Work out the finished part from the listing and answer in its coordinate system (mm). Coordinates: 2 decimals unless noted, no trailing zeros. Order: outer loops, then holes, each group sorted by start corner. A loop starts at its lowest first (then second) coordinate and runs counter-clockwise, first axis right, second up.
1. Find the intervals of material crossed by probe 1 along Y at (x, z) = (6.5, 10.5); probe 2 along Y at (x, z) = (0, 43); probe 3 along Y at (x, z) = (8.5, 6), in increasing order.
2. Flat-ended cylindrical pins translate along their axes: pin 1 Ø6 at (y, z) = (-10.5, 67) entering from -X; pin 2 Ø12 at (x, z) = (2, 14) entering from -Y; pin 3 Ø0.7 at (x, z) = (-1.5, 45.5) entering from -Y. Find the tip coordinate at first contact, or state that the pin passes through.
3. The part is cut by section A-A, the plane y = -2. Give the vertices of the cut face in (x, z), then the cut area to 3 significant figures.
4. The part is cut by section B-B, the plane z = 72.5. Count the separate pieces of the cut face and the enclosed holes in it, then the cut area to 3 significant figures.
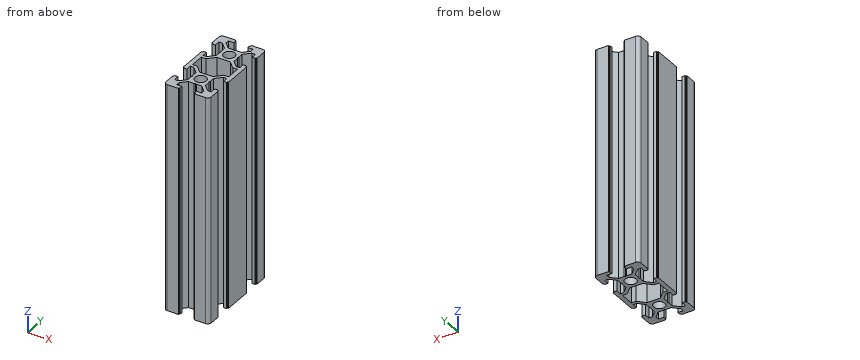
```python
from build123d import *

# Parameters (mm, degrees)
MODEL_R         = 2.5
EXTRUDE_1_DEPTH = 100


with BuildPart() as part:
    # Model → 凸台-拉伸1 (new body)
    with BuildSketch(Plane.XY):
        with BuildLine():
            Line((-3.6, 10), (-3.9, 9.480384758))
            Line((-3.9, 9.480384758), (-3.9, 7.089949494))
            Line((-3.9, 7.089949494), (-6.489949494, 4.5))
            Line((-6.489949494, 4.5), (-8.1, 4.5))
            Line((-8.1, 4.5), (-8.1, 6.9))
            Line((-8.1, 6.9), (-9.5, 6.9))
            Line((-9.5, 6.9), (-9.5, 6.4))
            Line((-9.5, 6.4), (-10, 6.4))
            Line((-10, 6.4), (-10, -6.4))
            Line((-10, -6.4), (-9.5, -6.4))
            Line((-9.5, -6.4), (-9.5, -6.9))
            Line((-9.5, -6.9), (-8.1, -6.9))
            Line((-8.1, -6.9), (-8.1, -4.5))
            Line((-8.1, -4.5), (-6.489949494, -4.5))
            Line((-6.489949494, -4.5), (-3.9, -7.089949494))
            Line((-3.9, -7.089949494), (-3.9, -9.480384758))
            Line((-3.9, -9.480384758), (-3.6, -10))
            Line((-3.6, -10), (-3.9, -10.519615242))
            Line((-3.9, -10.519615242), (-3.9, -12.910050506))
            Line((-3.9, -12.910050506), (-6.489949494, -15.5))
            Line((-6.489949494, -15.5), (-8.1, -15.5))
            Line((-8.1, -15.5), (-8.1, -13.1))
            Line((-8.1, -13.1), (-9.5, -13.1))
            Line((-9.5, -13.1), (-9.5, -13.6))
            Line((-9.5, -13.6), (-10, -13.6))
            Line((-10, -13.6), (-10, -18.5))
            ThreePointArc((-10, -18.5), (-9.560660172, -19.560660172), (-8.5, -20))
            Line((-8.5, -20), (-3.6, -20))
            Line((-3.6, -20), (-3.6, -19.5))
            Line((-3.6, -19.5), (-3.1, -19.5))
            Line((-3.1, -19.5), (-3.1, -18.1))
            Line((-3.1, -18.1), (-5.5, -18.1))
            Line((-5.5, -18.1), (-5.5, -16.489949494))
            Line((-5.5, -16.489949494), (-2.910050506, -13.9))
            Line((-2.910050506, -13.9), (-0.519615242, -13.9))
            Line((-0.519615242, -13.9), (0, -13.6))
            Line((0, -13.6), (0.519615242, -13.9))
            Line((0.519615242, -13.9), (2.910050506, -13.9))
            Line((2.910050506, -13.9), (5.5, -16.489949494))
            Line((5.5, -16.489949494), (5.5, -18.1))
            Line((5.5, -18.1), (3.1, -18.1))
            Line((3.1, -18.1), (3.1, -19.5))
            Line((3.1, -19.5), (3.6, -19.5))
            Line((3.6, -19.5), (3.6, -20))
            Line((3.6, -20), (8.5, -20))
            ThreePointArc((8.5, -20), (9.560660172, -19.560660172), (10, -18.5))
            Line((10, -18.5), (10, -13.6))
            Line((10, -13.6), (9.5, -13.6))
            Line((9.5, -13.6), (9.5, -13.1))
            Line((9.5, -13.1), (8.1, -13.1))
            Line((8.1, -13.1), (8.1, -15.5))
            Line((8.1, -15.5), (6.489949494, -15.5))
            Line((6.489949494, -15.5), (3.9, -12.910050506))
            Line((3.9, -12.910050506), (3.9, -10.519615242))
            Line((3.9, -10.519615242), (3.6, -10))
            Line((3.6, -10), (3.9, -9.480384758))
            Line((3.9, -9.480384758), (3.9, -7.089949494))
            Line((3.9, -7.089949494), (6.489949494, -4.5))
            Line((6.489949494, -4.5), (8.1, -4.5))
            Line((8.1, -4.5), (8.1, -6.9))
            Line((8.1, -6.9), (9.5, -6.9))
            Line((9.5, -6.9), (9.5, -6.4))
            Line((9.5, -6.4), (10, -6.4))
            Line((10, -6.4), (10, 6.4))
            Line((10, 6.4), (9.5, 6.4))
            Line((9.5, 6.4), (9.5, 6.9))
            Line((9.5, 6.9), (8.1, 6.9))
            Line((8.1, 6.9), (8.1, 4.5))
            Line((8.1, 4.5), (6.489949494, 4.5))
            Line((6.489949494, 4.5), (3.9, 7.089949494))
            Line((3.9, 7.089949494), (3.9, 9.480384758))
            Line((3.9, 9.480384758), (3.6, 10))
            Line((3.6, 10), (3.9, 10.519615242))
            Line((3.9, 10.519615242), (3.9, 12.910050506))
            Line((3.9, 12.910050506), (6.489949494, 15.5))
            Line((6.489949494, 15.5), (8.1, 15.5))
            Line((8.1, 15.5), (8.1, 13.1))
            Line((8.1, 13.1), (9.5, 13.1))
            Line((9.5, 13.1), (9.5, 13.6))
            Line((9.5, 13.6), (10, 13.6))
            Line((10, 13.6), (10, 18.5))
            ThreePointArc((10, 18.5), (9.560660172, 19.560660172), (8.5, 20))
            Line((8.5, 20), (3.6, 20))
            Line((3.6, 20), (3.6, 19.5))
            Line((3.6, 19.5), (3.1, 19.5))
            Line((3.1, 19.5), (3.1, 18.1))
            Line((3.1, 18.1), (5.5, 18.1))
            Line((5.5, 18.1), (5.5, 16.489949494))
            Line((5.5, 16.489949494), (2.910050506, 13.9))
            Line((2.910050506, 13.9), (0.519615242, 13.9))
            Line((0.519615242, 13.9), (0, 13.6))
            Line((0, 13.6), (-0.519615242, 13.9))
            Line((-0.519615242, 13.9), (-2.910050506, 13.9))
            Line((-2.910050506, 13.9), (-5.5, 16.489949494))
            Line((-5.5, 16.489949494), (-5.5, 18.1))
            Line((-5.5, 18.1), (-3.1, 18.1))
            Line((-3.1, 18.1), (-3.1, 19.5))
            Line((-3.1, 19.5), (-3.6, 19.5))
            Line((-3.6, 19.5), (-3.6, 20))
            Line((-3.6, 20), (-8.5, 20))
            ThreePointArc((-8.5, 20), (-9.560660172, 19.560660172), (-10, 18.5))
            Line((-10, 18.5), (-10, 13.6))
            Line((-10, 13.6), (-9.5, 13.6))
            Line((-9.5, 13.6), (-9.5, 13.1))
            Line((-9.5, 13.1), (-8.1, 13.1))
            Line((-8.1, 13.1), (-8.1, 15.5))
            Line((-8.1, 15.5), (-6.489949494, 15.5))
            Line((-6.489949494, 15.5), (-3.9, 12.910050506))
            Line((-3.9, 12.910050506), (-3.9, 10.519615242))
            Line((-3.9, 10.519615242), (-3.6, 10))
        make_face()
        with Locations((0, 10)):
            Circle(MODEL_R, mode=Mode.SUBTRACT)
        with Locations((0, -10)):
            Circle(MODEL_R, mode=Mode.SUBTRACT)
        Polygon((8, -3.1), (5.910050506, -3.1), (2.910050506, -6.1), (-2.910050506, -6.1), (-5.910050506, -3.1), (-8, -3.1), (-8, 3.1), (-5.910050506, 3.1), (-2.910050506, 6.1), (2.910050506, 6.1), (5.910050506, 3.1), (8, 3.1), align=None, mode=Mode.SUBTRACT)
    extrude(amount=EXTRUDE_1_DEPTH)


solid = part.part
```
Geometry says:
1. probe 1: y = -20 to -15.5, -4.5 to -3.1, 3.1 to 4.5, 15.5 to 20
1. probe 2: y = -13.6 to -12.5, -7.5 to -6.1, 6.1 to 7.5, 12.5 to 13.6
1. probe 3: y = -20 to -13.1, -6.9 to 6.9, 13.1 to 20
2. pin 1: stops at x = -9.5
2. pin 2: stops at y = -20
2. pin 3: stops at y = -13.9
3. outline: (-10, 0) - (-8, 0) - (-8, 100) - (-10, 100) - close; (8, 0) - (10, 0) - (10, 100) - (8, 100) - close
3. area: 400 mm2
4. separate pieces: 1
4. enclosed holes: 3
4. area: 295 mm2
